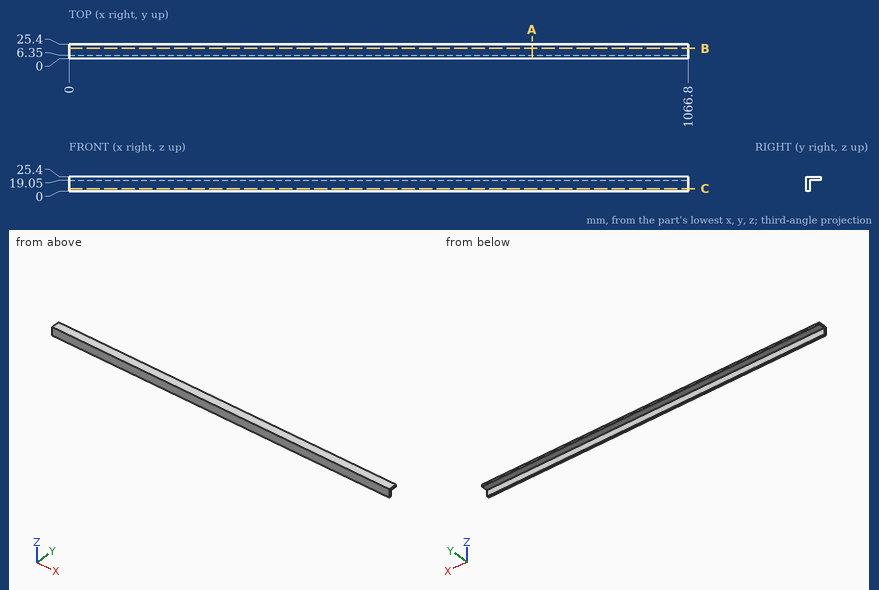
Source: three-view drawing plus pictorial views. Frame: mm from the lowest corner of the part. Coordinates: 2 decimals unless noted, no trailing zeros. Order: outer loops, then holes, each group sorted by start corner. A loop starts at its lowest first (then second) coordinate and runs counter-clockwise, first axis right, second up. Notation, with made-up numbers: (4, -0.5) -> (24, -0.5) arc R28 cw to (24, 27.5) -> close; hole circle Ø2 at (25.25, -11.5). An arc over 180 degrees is marked (long way). Write item = value, one per line.
(1) Cut plane A-A on x = 798. Return loops of the section in (y, z).
Solved:
outline = (0, 0) -> (6.35, 0) -> (6.35, 19.05) -> (25.4, 19.05) -> (25.4, 25.4) -> (0, 25.4) -> close
(2) Cut plane B-B on y = 17.75. Return loops of the section in (x, z).
Solved:
outline = (0, 19.05) -> (1066.8, 19.05) -> (1066.8, 25.4) -> (0, 25.4) -> close
(3) Pin query (flat end, axial travel): pin 1 Ø1 at (x, y) = (583, 11) entering from -Z; pin 2 Ø15 at (x, z) = (439.5, 10) entering from +Y. Return the tip coordinate at first contact, or that it passes through.
Solved:
pin_1 = 19.05
pin_2 = 6.35
(4) Line query: line 1 (Y direction, x = 598.5, z = 13); line 2 (Z direction, x = 447, y = 16). Output: solid intervals per line, ascending.
Solved:
line_1 = 0 to 6.35
line_2 = 19.05 to 25.4
(5) Cut plane C-C on z = 5. Return loops of the section in (x, y).
Solved:
outline = (0, 0) -> (1066.8, 0) -> (1066.8, 6.35) -> (0, 6.35) -> close
